```python
from build123d import *

# Parameters (mm, degrees)
ESQUISSE1_R             = 4.5
ESQUISSE1_R_2           = 2.6
EXTRUSION1_DEPTH        = 54.5
ESQUISSE2_OUTSIDE_W     = 32.948
ESQUISSE2_OUTSIDE_H     = 32.948
ESQUISSE2_OUTSIDE_R     = 4
ENL_V_MAT_EXTRU_1_DEPTH = 20
CHANFREIN1_SIZE         = 1


with BuildPart() as part:
    # Esquisse1 → Extrusion1 (new body, symmetric)
    with BuildSketch(Plane(origin=(0, 0, 0), x_dir=(0, 0, -1), z_dir=(1, 0, 0))):
        Circle(ESQUISSE1_R)
        Circle(ESQUISSE1_R_2, mode=Mode.SUBTRACT)
    extrude(amount=EXTRUSION1_DEPTH, both=True)

    # Esquisse2 outside → Enlèv. mat.-Extru.1 (cut, symmetric)
    with BuildSketch(Plane(origin=(0, 0, 0), x_dir=(0, 0, -1), z_dir=(1, 0, 0))):
        Rectangle(ESQUISSE2_OUTSIDE_W, ESQUISSE2_OUTSIDE_H)
        Circle(ESQUISSE2_OUTSIDE_R, mode=Mode.SUBTRACT)
    extrude(amount=ENL_V_MAT_EXTRU_1_DEPTH, both=True, mode=Mode.SUBTRACT)

    # Chanfrein1
    chanfrein1_edges = [part.edges().sort_by_distance(p)[0] for p in [
        (-54.5, 0, 4.5),
        (54.5, 0, 4.5),
    ]]
    chamfer(chanfrein1_edges, length=CHANFREIN1_SIZE)


solid = part.part
```
Here's how the part is built. I have some questions about the finished solid (model axes, mm). A direction names the side the tool comes from. Give positions to 0.01 mm unless a question says otherwise; leave off trailing zeros. Write each loop counter-clockwise with the first axis right and the second up, starting at its lowest first coordinate (ties: lowest second). Pieces come first, ordered by that corner, then holes. Notation, with made-up numbers: M -27,49 L -4,49 A12 cw -4,60 Z; hole C 62,-33.75 d8. An arc over 180 degrees is marked long. Put each result on its own line as item: value. Start each with the question number.
Item 1: If we section it at D-D, the plane x = 6.5: Write out the boundary of the cut face in (y, z), then the cut area to 3 significant figures.
Item 2: Will these pins go through, and if not, where does the flat tip stop? pin 1 (5 mm diameter, centred on x = 3, z = 3.5, fed in from -Y); pin 2 (4.5 mm diameter, centred on y = 0, z = 0, fed in from +X).
Item 3: If we section it at A-A, the plane y = 0: Write out the boundary of the cut face in (x, z).
Item 4: If we section it at C-C, the plane x = -41.5: Write out the boundary of the cut face in (y, z), then the cut area to 3 significant figures.
Item 5: Thinking about a two-plate mould opening in Y: for faces 3 (the flat face through (-20, -3, 3)), 4 (the conical face through (54, 0, 4)), 5 (the cylindrical face through (-0.763, 2.578, 0.338)), which applies, +Y half, -Y half, draft (parallel to the pull), parting line (faces both ways), or undercut?
Item 6: I need wall thicknesses on L1, parallel to Y at x = 9, z = 0; L2, parallel to Y at x = 36, z = 0; L3, parallel to Z at x = -42, y = -1.75. Which ranges of each line are inside material? Lowest first, please. Write a range as from..to.
Item 7: On a 3-axis mill with a long thin cutter (end or side, diameter ignored), from which of +Z, -Z, +X, -X, +Y, -Y can I reach the whole of each face in a straight line? I mean faces 1 (the cylindrical face through (-36.52, 4.46, 0.59)), 2 (the cylindrical face through (-0.28, -3.905, 0.867)). Say none if no direction works.
Values:
1. outline: C 0,0 d8; hole C 0,0 d5.2
1. area: 29.0 mm²
2. pin 1: y = -3.87
2. pin 2: through
3. outline: M -54.5,-3.5 L -53.5,-4.5 L -20,-4.5 L -20,-4 L 20,-4 L 20,-4.5 L 53.5,-4.5 L 54.5,-3.5 L 54.5,-2.6 L -54.5,-2.6 Z; M -54.5,2.6 L 54.5,2.6 L 54.5,3.5 L 53.5,4.5 L 20,4.5 L 20,4 L -20,4 L -20,4.5 L -53.5,4.5 L -54.5,3.5 Z
4. outline: C 0,0 d9; hole C 0,0 d5.2
4. area: 42.4 mm²
5. face 3: draft
5. face 4: parting line
5. face 5: undercut
6. L1: -4..-2.6, 2.6..4
6. L2: -4.5..-2.6, 2.6..4.5
6. L3: -4.15..-1.92, 1.92..4.15
7. face 1: +X, -X
7. face 2: none
